from build123d import *

# Parameters (mm, degrees)
SKETCH1_R           = 21
SKETCH1_R_2         = 20
BOSS_EXTRUDE1_DEPTH = 3.5
SKETCH2_R           = 3.55
SKETCH2_R_2         = 6.55
SKETCH2_R_3         = 2.55
SKETCH2_R_4         = 8.5
SKETCH2_W           = 11.2
SKETCH2_H           = 4.84
BOSS_EXTRUDE2_DEPTH = 5
SKETCH3_W           = 11.2
SKETCH3_H           = 4.84
SKETCH3_W_2         = 49
SKETCH3_H_2         = 8
SKETCH3_R           = 8.5
IGNORE_DEPTH        = 5
SKETCH4_R           = 8.5
SKETCH4_W           = 11.2
SKETCH4_H           = 4.84
CUT_EXTRUDE2_DEPTH  = 71.901339903
FILLET1_R           = 3
SKETCH5_W           = 42
SKETCH5_H           = 3.5
CUT_EXTRUDE3_DEPTH  = 25
CUT_EXTRUDE5_DEPTH  = 10
FILLET2_R           = 3
SKETCH8_R           = 1
CUT_EXTRUDE6_DEPTH  = 20


with BuildPart() as part:
    # Sketch1 → Boss-Extrude1 (new body)
    with BuildSketch(Plane(origin=(0, 0, 0), x_dir=(1, 0, 0), z_dir=(0, 1, 0))):
        with Locations(Location((0, 0, 0), (0, 0, 90))):
            Circle(SKETCH1_R)
        with Locations(Location((0, 0, 0), (0, 0, 90))):
            Circle(SKETCH1_R_2, mode=Mode.SUBTRACT)
    extrude(amount=BOSS_EXTRUDE1_DEPTH)

    # Sketch2 → Boss-Extrude2 (add)
    with BuildSketch(Plane(origin=(0, 3.5, 0), x_dir=(1, 0, 0), z_dir=(0, 1, 0))):
        Polygon((-29, -5), (-29, -29), (29, -29), (29, -5), (39, -5), (39, 5), (29, 5), (29, 29), (24.5, 29), (24.5, 51), (-24.5, 51), (-24.5, 29), (-29, 29), (-29, 5), (-39, 5), (-39, -5), align=None)
        with Locations(Location((-23.55, -23.55, 0), (0, 0, 270))):
            Circle(SKETCH2_R, mode=Mode.SUBTRACT)
        with Locations(Location((23.55, -23.55, 0), (0, 0, 270))):
            Circle(SKETCH2_R, mode=Mode.SUBTRACT)
        with Locations(Location((0, 0, 0), (0, 0, 270))):
            Circle(SKETCH2_R_2, mode=Mode.SUBTRACT)
        with Locations(Location((-23.55, 23.55, 0), (0, 0, 270))):
            Circle(SKETCH2_R, mode=Mode.SUBTRACT)
        with Locations(Location((23.55, 23.55, 0), (0, 0, 270))):
            Circle(SKETCH2_R, mode=Mode.SUBTRACT)
        with Locations(Location((-34, 0, 0), (0, 0, 270))):
            Circle(SKETCH2_R_3, mode=Mode.SUBTRACT)
        with Locations(Location((34, 0, 0), (0, 0, 270))):
            Circle(SKETCH2_R_3, mode=Mode.SUBTRACT)
        with Locations(Location((13.76, 39, 0), (0, 0, 270))):
            Circle(SKETCH2_R_4, mode=Mode.SUBTRACT)
        with Locations(Location((-13.76, 39, 0), (0, 0, 270))):
            Circle(SKETCH2_R_4, mode=Mode.SUBTRACT)
        with Locations((0, 46.28)):
            Rectangle(SKETCH2_W, SKETCH2_H, mode=Mode.SUBTRACT)
    extrude(amount=BOSS_EXTRUDE2_DEPTH)

    # Sketch3 → Ignore (add)
    with BuildSketch(Plane(origin=(0, 3.5, 0), x_dir=(1, 0, 0), z_dir=(0, 1, 0))):
        with Locations((0, 46.28)):
            Rectangle(SKETCH3_W, SKETCH3_H)
        with Locations((0, 55)):
            Rectangle(SKETCH3_W_2, SKETCH3_H_2)
        with Locations((13.76, 39)):
            Circle(SKETCH3_R)
        with Locations((-13.76, 39)):
            Circle(SKETCH3_R)
    extrude(amount=IGNORE_DEPTH)

    # Sketch4 → Cut-Extrude2 (cut, through all)
    with BuildSketch(Plane(origin=(0, 3.5, 0), x_dir=(1, 0, 0), z_dir=(0, 1, 0))):
        with Locations(Location((-13.75, 48, 0), (0, 0, 270))):
            Circle(SKETCH4_R)
        with Locations(Location((13.75, 48, 0), (0, 0, 270))):
            Circle(SKETCH4_R)
        with Locations((-0.079148889, 40.42)):
            Rectangle(SKETCH4_W, SKETCH4_H)
    extrude(amount=CUT_EXTRUDE2_DEPTH, mode=Mode.SUBTRACT)

    # Fillet1
    fillet1_edges = [part.edges().sort_by_distance(p)[0] for p in [
        (-29, 6, 29),
        (29, 6, 29),
        (39, 6, 5),
        (39, 6, -5),
        (29, 6, -29),
        (-29, 6, -29),
        (-39, 6, -5),
        (-39, 6, 5),
        (24.5, 6, -59),
        (-24.5, 6, -59),
    ]]
    fillet(fillet1_edges, radius=FILLET1_R)

    # Sketch5 → Cut-Extrude3 (cut, symmetric)
    with BuildSketch(Plane.XY):
        with Locations((0, 1.75)):
            Rectangle(SKETCH5_W, SKETCH5_H)
    extrude(amount=CUT_EXTRUDE3_DEPTH, both=True, mode=Mode.SUBTRACT)

    # Sketch6 → Cut-Extrude5 (cut)
    with BuildSketch(Plane(origin=(0, 8.5, 0), x_dir=(1, 0, 0), z_dir=(0, 1, 0))):
        Polygon((-26, 29), (24.5, 29), (43.321910497, 29), (43.321910497, -33.14300085), (-52.072842779, -33.14300085), (-52.072842779, 29), (-38.2971121, 29), align=None)
    extrude(amount=-CUT_EXTRUDE5_DEPTH, mode=Mode.SUBTRACT)

    # Fillet2
    fillet2_edges = [part.edges().sort_by_distance(p)[0] for p in [
        (24.5, 6, -29),
        (-24.5, 6, -29),
    ]]
    fillet(fillet2_edges, radius=FILLET2_R)

    # Sketch8 → Cut-Extrude6 (cut)
    with BuildSketch(Plane.XZ.offset(-3.5)):
        with Locations(Location((-21.329148889, -39.25, 0), (0, 0, 270))):
            Circle(SKETCH8_R)
        with Locations(Location((-21.329148889, -56.75, 0), (0, 0, 270))):
            Circle(SKETCH8_R)
        with Locations(Location((21.170851111, -56.75, 0), (0, 0, 270))):
            Circle(SKETCH8_R)
        with Locations(Location((21.170851111, -39.25, 0), (0, 0, 270))):
            Circle(SKETCH8_R)
    extrude(amount=-CUT_EXTRUDE6_DEPTH, mode=Mode.SUBTRACT)


solid = part.part
Design review of the part built by this model. Coordinates are the model's own, in mm. A direction names the side the tool comes from. Coordinates: 2 decimals unless noted, no trailing zeros. Loops run counter-clockwise (first coordinate to the right, second up) from the corner with the lowest first, then second, coordinate; pieces in that order, holes last. Notation, with made-up numbers: (-15, 57.5) - (43, 57.5) arc R5 cw to (43, 61.5) - close; hole circle Ø11 at (-0.75, 39). An arc over 180 degrees is marked (long way). Use CSV: the item, a comma, the result in double quotes. Start each with the question number.
1. Add section B-B on z = -48. Give the boundary of the cut face in (x, y).
2. For faces 4 (the flat face through (-24.5, 6, -44)), 5 (the flat face through (0, 6, -42.84)), list the 3-axis set-ups (+Z, -Z, +X, -X, +Y, -Y) from which the entire face can be reached by the end or side of a thin tool; tool diameter is ignored.
3. To check wall thickness, follow probe 1 along X at (y, z) = (7.55, -39.25); probe 2 along X at (y, z) = (6.65, -48); probe 3 along X at (y, z) = (4.8, -56.75). State the ranges of each line that lie inside material, in increasing order.
4. Add section D-D on x = 13.75. Give the boundary of the cut face in (y, z).
5. Mouldability with a two-part tool opening along Z and no side actions: class faces 1 (the cylindrical face through (-22.216, 5.965, -39.711)), 2 (the flat face through (0, 8.5, -44)), 3 (the flat face through (0, 6, -29)) as released by +Z, released by -Z, zero draft, split by the parting line, or undercut.
6. Add section A-A on x = -1. Give the boundary of the cut face in (y, z).
7. Add section C-C on y = 4.1. Give the boundary of the cut face in (x, z), plus the area to 3 significant figures.
Resolved:
1,outline,"(-24.5, 3.5) - (-22.25, 3.5) - (-22.25, 8.5) - (-24.5, 8.5) - close; (-5.25, 3.5) - (5.25, 3.5) - (5.25, 8.5) - (-5.25, 8.5) - close; (22.25, 3.5) - (24.5, 3.5) - (24.5, 8.5) - (22.25, 8.5) - close"
2,face 4,"+Z, -Z, -X, +Y, -Y"
2,face 5,"+Y, -Y"
3,probe 1,"-24.5 to -22.33, -20.33 to -5.68, 5.52 to 20.17, 22.17 to 24.5"
3,probe 2,"-24.5 to -22.25, -5.25 to 5.25, 22.25 to 24.5"
3,probe 3,"-24.4 to -22.33, -20.33 to 20.17, 22.17 to 24.4"
4,outline,"(3.5, -59) - (8.5, -59) - (8.5, -56.5) - (3.5, -56.5) - close; (3.5, -39.5) - (8.5, -39.5) - (8.5, -29) - (3.5, -29) - close"
5,face 1,"undercut"
5,face 2,"zero draft"
5,face 3,"released by +Z"
6,outline,"(3.5, -59) - (8.5, -59) - (8.5, -42.84) - (3.5, -42.84) - close; (3.5, -38) - (8.5, -38) - (8.5, -29) - (3.5, -29) - close"
7,outline,"(-24.5, -56) arc R3 ccw to (-21.5, -59) - (21.5, -59) arc R3 ccw to (24.5, -56) - (24.5, -32) arc R3 ccw to (21.5, -29) - (-21.5, -29) arc R3 ccw to (-24.5, -32) - close; hole circle Ø2 at (-21.33, -56.75); hole circle Ø2 at (-21.33, -39.25); hole circle Ø17 at (-13.75, -48); hole (-5.68, -42.84) - (5.52, -42.84) - (5.52, -38) - (-5.68, -38) - close; hole circle Ø17 at (13.75, -48); hole circle Ø2 at (21.17, -56.75); hole circle Ø2 at (21.17, -39.25)"
7,area,"942 mm2"
